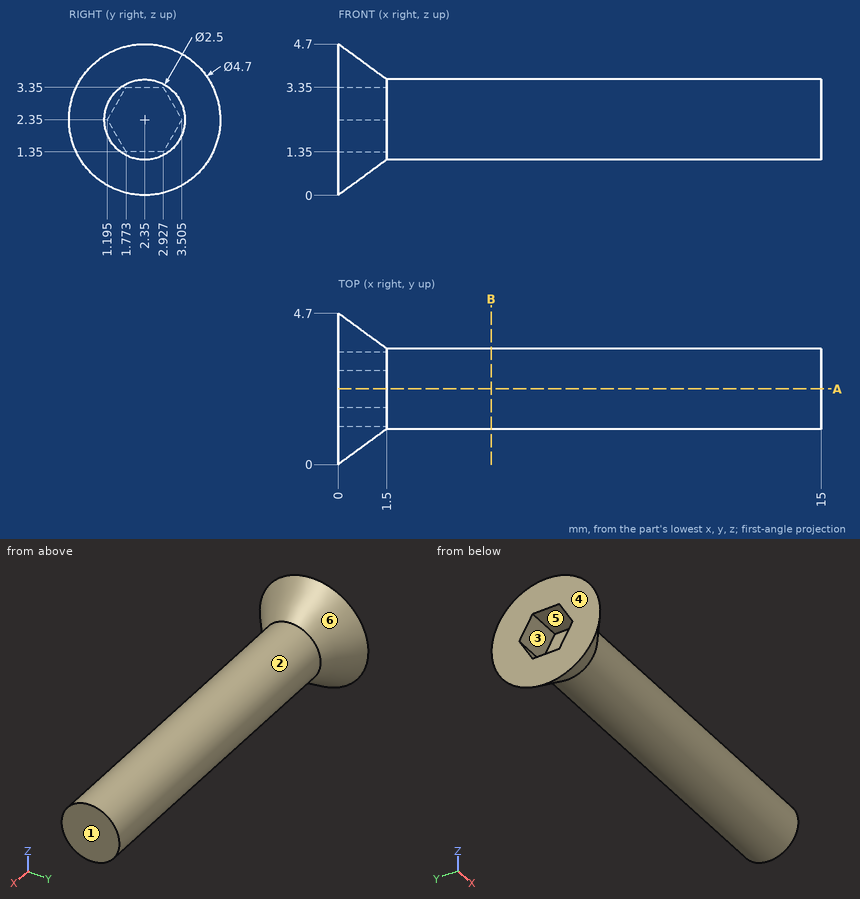
Geometry check sheet. Reference: drawing and pictorial views, mm from the part's lowest x, y, z. A direction names the side the tool comes from. Round coordinates to 2 decimals unless told otherwise and drop trailing zeros. Loops run counter-clockwise (first coordinate to the right, second up) from the corner with the lowest first, then second, coordinate; pieces in that order, holes last. Notation, with made-up numbers: (71.25, 30) - (75.25, 30) arc R28 cw to (75.25, 56) - close; hole circle Ø8 at (10, -28). An arc over 180 degrees is marked (long way). Answer in a Markdown table with one row per item. Add a question column.
Q1. Section check A-A on y = 2.35. Enter the section's corners in (x, z).
Q2. Gauge pin test, flat ends, axial feed: pin 1 (0.9 mm diameter, centred on x = 1, y = 2.5, fed in from +Z); pin 2 (1 mm diameter, centred on y = 2, z = 2.5, fed in from -X); pin 3 (1.5 mm diameter, centred on x = 7, y = 2.5, fed in from +Z). Record the tip position at first contact, or that the pin passes through.
Q3. Tool access check on the marked faces 1 and 2. Record the directions out of +Z, -Z, +X, -X, +Y, -Y that give a thin tool (end or side, any length) a straight path to the whole face; none if there is none.
Q4. Section check B-B on x = 4.75. Enter the section's corners in (y, z).
Q5. Release check for a two-part mould opening along Z. For the marked faces 3, 4, 5 and 6 record: pulls with the +Z half, pulls with the -Z half, needs draft (parallel to the pull), parting line crosses it, or undercut.
Q6. Material ranges on line 1 (Y direction, x = 11, z = 2.3); line 2 (X direction, y = 2.15, z = 1.85), recorded low to high.
Found:
| question | item | result |
|---|---|---|
| 1 | outline | (0, 0) - (1.5, 1.1) - (15, 1.1) - (15, 3.6) - (1.5, 3.6) - (0, 4.7) - (0, 3.35) - (1.5, 3.35) - (1.5, 1.35) - (0, 1.35) - close |
| 2 | pin 1 | stops at z = 4.29 |
| 2 | pin 2 | stops at x = 1.5 |
| 2 | pin 3 | stops at z = 3.6 |
| 3 | face 1 | +Z, -Z, +X, +Y, -Y |
| 3 | face 2 | +X |
| 4 | outline | circle Ø2.5 at (2.35, 2.35) |
| 5 | face 3 | undercut |
| 5 | face 4 | needs draft |
| 5 | face 5 | undercut |
| 5 | face 6 | parting line crosses it |
| 6 | line 1 | y = 1.1 to 3.6 |
| 6 | line 2 | x = 1.5 to 15 |
